```python
from build123d import *

# Parameters (mm, degrees)
BOSS_EXTRU_1_DEPTH      = 235
ESQUISSE2_R             = 44.45
ENL_V_MAT_EXTRU_1_DEPTH = 78
ESQUISSE3_R             = 28.575
ENL_V_MAT_EXTRU_2_DEPTH = 199.597583067
BOSS_EXTRU_4_DEPTH      = 33
ESQUISSE8_W             = 33
ESQUISSE8_H             = 90
ENL_V_MAT_EXTRU_4_DEPTH = 19
ENL_V_MAT_EXTRU_5_DEPTH = 13


with BuildPart() as part:
    # Esquisse1 → Boss.-Extru.1 (new body)
    with BuildSketch(Plane.XY):
        with BuildLine():
            Line((0, -86), (0, 86))
            ThreePointArc((0, 86), (-60.811183182, 60.811183182), (-86, 0))
            Line((-86, 0), (-86, -43.853430349))
            Line((-86, -43.853430349), (-13, -86))
            Line((-13, -86), (0, -86))
        make_face()
    extrude(amount=BOSS_EXTRU_1_DEPTH)

    # Esquisse2 → Enlèv. mat.-Extru.1 (cut)
    with BuildSketch(Plane.XY.offset(235)):
        Circle(ESQUISSE2_R)
    extrude(amount=-ENL_V_MAT_EXTRU_1_DEPTH, mode=Mode.SUBTRACT)

    # Esquisse3 → Enlèv. mat.-Extru.2 (cut, through all)
    with BuildSketch(Plane.XY.offset(157)):
        Circle(ESQUISSE3_R)
    extrude(amount=-ENL_V_MAT_EXTRU_2_DEPTH, mode=Mode.SUBTRACT)

    # Esquisse7 → Boss.-Extru.4 (add)
    with BuildSketch(Plane.XY.offset(235)):
        with BuildLine():
            Line((-64.719928969, 0), (-40.188548434, 31.398735242))
            Line((-40.188548434, 31.398735242), (-14.235687992, 64.616881796))
            Line((-14.235687992, 64.616881796), (-33.116437077, 79.368139674))
            ThreePointArc((-33.116437077, 79.368139674), (-66.952455175, 53.975631039), (-84.587575845, 15.522306937))
            Line((-84.587575845, 15.522306937), (-64.719928969, 0))
        make_face()
    extrude(amount=BOSS_EXTRU_4_DEPTH)

    # Esquisse8 → Enlèv. mat.-Extru.4 (cut)
    with BuildSketch(Plane(origin=(0, 0, 0), x_dir=(0, 0, -1), z_dir=(1, 0, 0))):
        with Locations((-54.5, 49.335999727)):
            Rectangle(ESQUISSE8_W, ESQUISSE8_H)
    extrude(amount=-ENL_V_MAT_EXTRU_4_DEPTH, mode=Mode.SUBTRACT)

    # Esquisse9 → Enlèv. mat.-Extru.5 (cut)
    with BuildSketch(Plane(origin=(0, 0, 0), x_dir=(0, 0, -1), z_dir=(1, 0, 0))):
        with BuildLine():
            Line((-110, -49), (0, -49))
            Line((0, -49), (0, -71))
            Line((0, -71), (-110, -71))
            ThreePointArc((-110, -71), (-121, -60), (-110, -49))
        make_face()
    extrude(amount=-ENL_V_MAT_EXTRU_5_DEPTH, mode=Mode.SUBTRACT)


solid = part.part
```
Source: CAD feature listing. Evaluate the final solid. Frame: model axes, mm. A direction names the side the tool comes from. Round coordinates to 2 decimals unless told otherwise and drop trailing zeros. Loops run counter-clockwise (first coordinate to the right, second up) from the corner with the lowest first, then second, coordinate; pieces in that order, holes last. Notation, with made-up numbers: M 2,42 L 16,42 A30 cw 16,70 Z; hole C -28.5,-27 d3. An arc over 180 degrees is marked long. Use a Markdown table: item, result. Add a question column.
1. Set-up query: faces 1 (the flat face through (-19, 53, 55)), 2 (the flat face through (-23.544, 71.889, 251.269)), 3 (the flat face through (-32, 1, 157)). Return all of +Z, -Z, +X, -X, +Y, -Y with unobstructed straight access to the full face (end or side cutting, diameter ignored); none if empty.
2. Pull-direction query (Y, two-part tool) for faces 4 (the flat face through (-50, 40, 268)), 5 (the flat face through (-74.79, 7.87, 251.27)), 6 (the flat face through (-6, -71, 54)), 7 (the cylindrical face through (-6, -60, 121)); classes: +Y half, -Y half, draft (parallel to the pull), parting line (faces both ways), or undercut.
3. Cut plane B-B, the plane y = 39. Output: boundary loops of the cut face in (x, z), and give its area (3 significant figures).
4. Ray query, line 1 along Y through (x, z) = (-12, 87.5); line 2 along Y through (x, z) = (-8.5, 230.5); line 3 along X through (y, z) = (-1, 189). Return the intervals inside material, ascending. Write a range as [from, to].
5. Cut plane A-A, the plane z = 213.5. Output: boundary loops of the cut face in (x, y), and give its area (3 significant figures).
6. Contact query for flat-ended pins moving along their axis: pin 1 (5.5 mm diameter, centred on x = -12.5, y = 41, fed in from +Z); pin 2 (1 mm diameter, centred on y = 11.5, z = 147.5, fed in from -X); pin 3 (17.5 mm diameter, centred on y = -59, z = 30.5, fed in from +X). Output: stop coordinate, or through.
7. Cut plane D-D, the plane z = 24.5. Output: boundary loops of the cut face in (x, y) (3 decimals), and give its area (3 significant figures).
8. Cut plane C-C, the plane x = -78.5. Output: boundary loops of the cut face in (y, z).
Solution:
| question | item | result |
|---|---|---|
| 1 | face 1 | +X, +Y |
| 1 | face 2 | +Z, +X, +Y |
| 1 | face 3 | +Z, +X |
| 2 | face 4 | draft |
| 2 | face 5 | -Y half |
| 2 | face 6 | undercut |
| 2 | face 7 | undercut |
| 3 | outline | M -76.65,0 L 0,0 L 0,38 L -19,38 L -19,71 L 0,71 L 0,157 L -21.33,157 L -21.33,235 L -34.25,235 L -34.25,268 L -76.65,268 Z |
| 3 | area | 17,100 mm2 |
| 4 | line 1 | y = [-86, -71], [-49, -25.93], [25.93, 85.16] |
| 4 | line 2 | y = [-86, -43.63], [43.63, 85.58] |
| 4 | line 3 | x = [-86, -44.44] |
| 5 | outline | M -86,-43.85 L -13,-86 L 0,-86 L 0,-44.45 A44.45 cw 0,44.45 L 0,86 A86 ccw -86,0 Z |
| 5 | area | 8,560 mm2 |
| 6 | pin 1 | stops at z = 235 |
| 6 | pin 2 | stops at x = -85.29 |
| 6 | pin 3 | stops at x = -13 |
| 7 | outline | M -86,-43.853 L -13,-86 L 0,-86 L 0,-71 L -13,-71 L -13,-49 L 0,-49 L 0,-28.575 A28.575 cw 0,28.575 L 0,86 A86 ccw -86,0 Z |
| 7 | area | 10,100 mm2 |
| 8 | outline | M -48.18,0 L 35.12,0 L 35.12,268 L 10.77,268 L 10.77,235 L -48.18,235 Z |
